from build123d import *

# Parameters (mm, degrees)
SKETCH1_W                                = 53.2
SKETCH1_H                                = 134.9
SKETCH1_R                                = 1.25
BOSS_EXTRUDE1_DEPTH                      = 3.5
POLOLU_MOUNTING_BRACKET_R                = 2
POLOLU_37MM_MOUNTING_BRACKET_HOLES_DEPTH = 146.053438429


with BuildPart() as part:
    # Sketch1 → Boss-Extrude1 (new body)
    with BuildSketch(Plane(origin=(0, 0, 0), x_dir=(1, 0, 0), z_dir=(0, 1, 0))):
        with Locations((-26.6, 67.45)):
            Rectangle(SKETCH1_W, SKETCH1_H)
        with Locations(Location((-50.7, 104.9, 0), (0, 0, 270))):
            Circle(SKETCH1_R, mode=Mode.SUBTRACT)
        with Locations(Location((-2.5, 111.05, 0), (0, 0, 270))):
            Circle(SKETCH1_R, mode=Mode.SUBTRACT)
        with Locations(Location((-35.5, 80.8, 0), (0, 0, 270))):
            Circle(SKETCH1_R, mode=Mode.SUBTRACT)
        with Locations(Location((-7.6, 80.8, 0), (0, 0, 270))):
            Circle(SKETCH1_R, mode=Mode.SUBTRACT)
        with Locations(Location((-50.7, 30, 0), (0, 0, 270))):
            Circle(SKETCH1_R, mode=Mode.SUBTRACT)
        with Locations(Location((-2.5, 28.7, 0), (0, 0, 270))):
            Circle(SKETCH1_R, mode=Mode.SUBTRACT)
    extrude(amount=BOSS_EXTRUDE1_DEPTH)

    # Pololu Mounting Bracket → Pololu 37mm mounting bracket holes (cut, through all)
    with BuildSketch(Plane(origin=(0, 3.5, 0), x_dir=(1, 0, 0), z_dir=(0, 1, 0))):
        with Locations(Location((-41.2, 4, 0), (0, 0, 270))):
            Circle(POLOLU_MOUNTING_BRACKET_R)
        with Locations(Location((-10, 4, 0), (0, 0, 270))):
            Circle(POLOLU_MOUNTING_BRACKET_R)
        with Locations(Location((-41.2, 42.4, 0), (0, 0, 270))):
            Circle(POLOLU_MOUNTING_BRACKET_R)
        with Locations(Location((-10, 42.4, 0), (0, 0, 270))):
            Circle(POLOLU_MOUNTING_BRACKET_R)
        with Locations(Location((-41.2, 130.9, 0), (0, 0, 90))):
            Circle(POLOLU_MOUNTING_BRACKET_R)
        with Locations(Location((-10, 130.9, 0), (0, 0, 90))):
            Circle(POLOLU_MOUNTING_BRACKET_R)
        with Locations(Location((-10, 92.5, 0), (0, 0, 90))):
            Circle(POLOLU_MOUNTING_BRACKET_R)
        with Locations(Location((-41.2, 92.5, 0), (0, 0, 90))):
            Circle(POLOLU_MOUNTING_BRACKET_R)
    extrude(amount=-POLOLU_37MM_MOUNTING_BRACKET_HOLES_DEPTH, mode=Mode.SUBTRACT)


solid = part.part
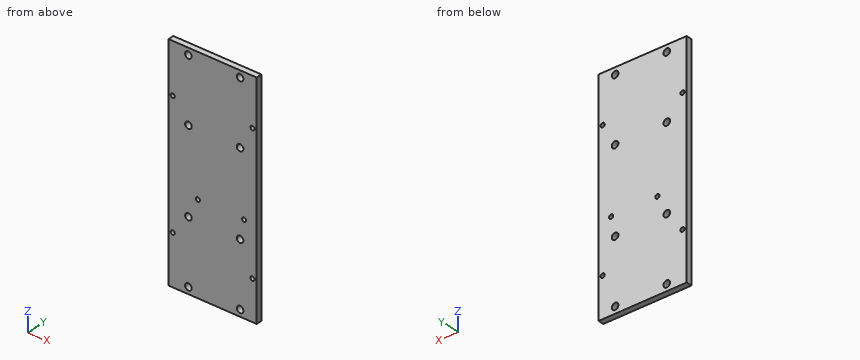
Model file for the job. Use its own axes, mm. Give positions to 0.01 mm unless a question says otherwise; leave off trailing zeros. Order: outer loops, then holes, each group sorted by start corner. A loop starts at its lowest first (then second) coordinate and runs counter-clockwise, first axis right, second up. Notation, with made-up numbers: M -27.5,30 L -19.5,30 A8 ccw -19.5,45 Z; hole C 15.25,89.5 d7. An arc over 180 degrees is marked long. Write item = value, one per line.
Q1. Cut at C-C, the plane x = -35.5. List the corners of the cut face in (y, z).
Derived:
outline = M 0,-134.9 L 3.5,-134.9 L 3.5,-82.05 L 0,-82.05 Z; M 0,-79.55 L 3.5,-79.55 L 3.5,0 L 0,0 Z
Q2. Drill centre lines: line 1 (X direction, y = 1.6, z = -4); line 2 (X direction, y = 2.05, z = -104.9); line 3 (X direction, y = 0.9, z = -80.8). Where is each one in solid material? Low to high. Write a range as [from, to].
Derived:
line_1 = [-53.2, -43.2], [-39.2, -12], [-8, 0]
line_2 = [-53.2, -51.95], [-49.45, 0]
line_3 = [-53.2, -36.75], [-34.25, -8.85], [-6.35, 0]
Q3. Flat gauge pin, fed straight in: pin 1 (3 mm diameter, centred on x = -10, z = -130.9, fed in from -Y). Where does the tip first touch, or does it go through?
Derived:
pin_1 = through
Q4. Cut at A-A, the plane z = -104.9. List the corners of the cut face in (x, y), then the cut area to 3 significant figures.
Derived:
outline = M -53.2,0 L -51.95,0 L -51.95,3.5 L -53.2,3.5 Z; M -49.45,0 L 0,0 L 0,3.5 L -49.45,3.5 Z
area = 177 mm2
Q5. Cut at D-D, the plane y = 0.75. Count the separate pieces of the cut face and the enclosed holes in it, then the cut area to 3 significant figures.
Derived:
separate_pieces = 1
enclosed_holes = 14
area = 7,050 mm2
Q6. Cut at B-B, the plane x = -50.7. List the corners of the cut face in (y, z), then the cut area to 3 significant figures.
Derived:
outline = M 0,-134.9 L 3.5,-134.9 L 3.5,-106.15 L 0,-106.15 Z; M 0,-103.65 L 3.5,-103.65 L 3.5,-31.25 L 0,-31.25 Z; M 0,-28.75 L 3.5,-28.75 L 3.5,0 L 0,0 Z
area = 455 mm2
